from build123d import *

# Parameters (mm, degrees)
F1_DEPTH = 130
F2_R     = 6
F3_DEPTH = 5.001
F4_R     = 5
F5_DEPTH = 111.001


with BuildPart() as f1:
    # F0 (on Top) → F1 (new body)
    with BuildSketch(Plane.XY):
        with BuildLine():
            Line((17.922193, 92.008901), (-54.077807, 92.008901))
            Line((-54.077807, 92.008901), (-54.077807, 87.008901))
            Line((-54.077807, 87.008901), (14.922193, 87.008901))
            ThreePointArc((14.922193, 87.008901), (17.043514, 86.130221), (17.922193, 84.008901))
            Line((17.922193, 84.008901), (17.922193, -10.991095))
            ThreePointArc((17.922193, -10.991095), (17.043514, -13.112415), (14.922193, -13.991095))
            Line((14.922193, -13.991095), (-54.077807, -13.991095))
            Line((-54.077807, -13.991095), (-54.077807, -18.991099))
            Line((-54.077807, -18.991099), (17.922193, -18.991099))
            ThreePointArc((17.922193, -18.991099), (21.457727, -17.526633), (22.922193, -13.991099))
            Line((22.922193, -13.991099), (22.922193, 87.008901))
            ThreePointArc((22.922193, 87.008901), (21.457727, 90.544435), (17.922193, 92.008901))
        make_face()
    extrude(amount=F1_DEPTH)

    # F2 (on face) → F3 (cut, through all)
    with BuildSketch(Plane(origin=(17.922193, 0, 0), x_dir=(0, -1, 0), z_dir=(-1, 0, 0))):
        with Locations((-15.887585, 105)):
            Circle(F2_R)
        with Locations((-36.508901, 25)):
            Circle(F2_R)
        with Locations((-58.008901, 105)):
            Circle(F2_R)
    extrude(amount=-F3_DEPTH, mode=Mode.SUBTRACT)

    # F4 (on face) → F5 (cut, through all)
    with BuildSketch(Plane(origin=(0, 92.008901, 0), x_dir=(-1, 0, 0), z_dir=(0, 1, 0))):
        with Locations((39.077807, 25)):
            Circle(F4_R)
        with Locations((4.077807, 25)):
            Circle(F4_R)
        Polygon((12.077807, 75), (54.077807, 30), (54.077807, 130), (-17.922193, 130), (-17.922193, 75), align=None)
    extrude(amount=-F5_DEPTH, mode=Mode.SUBTRACT)


solid = f1.part
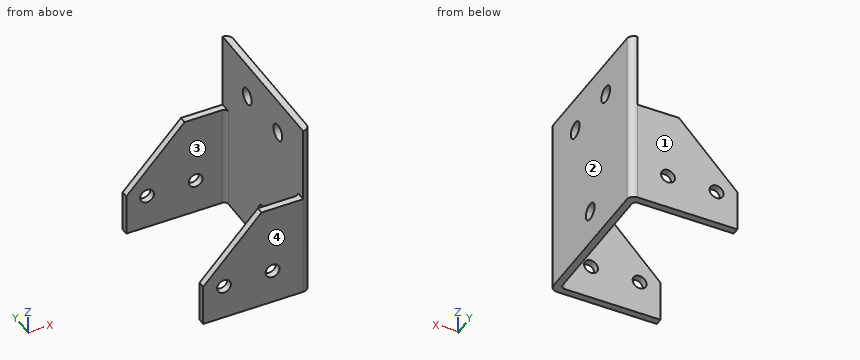
Could you check a few things on this model? Use its own coordinates, in mm. Face numbers are marked on the shaded views. Coordinates: 2 decimals unless noted, no trailing zeros. Write each loop counter-clockwise with the first axis right and the second up, starting at its lowest first coordinate (ties: lowest second). Pieces come first, ordered by that corner, then holes. Notation, with made-up numbers: M -15,58.5 L 43,58.5 A16 cw 43,67.5 Z; hole C 32,-7.5 d1. An arc over 180 degrees is marked long. One line per question, with ' | ' between items.
1) If we mould it in two halves opening along Y, with no side actions, what happens to the marked faces 1, 2, 3 and 4? For each: released by +Y, released by -Y, zero draft, split by the parting line, or undercut.
Checks:
face 1: released by +Y | face 2: zero draft | face 3: undercut | face 4: released by -Y
2) Imagine slicing it at A-A, the plane x = 7. Write out the boundary of the cut face in (y, z), and give its area (3 significant figures).
Checks:
outline: M -18.99,0 L -13.99,0 L -13.99,75 L -18.99,75 Z; M 87.01,0 L 92.01,0 L 92.01,75 L 87.01,75 Z | area: 750 mm²
3) I need wall thicknesses on probe 1 along Y at (x, z) = (2.5, 51.5); probe 2 along X at (y, z) = (-12, 121); probe 3 along X at (y, z) = (86, 52). Which ranges of each line are inside material? Lowest first, please. Write a range as [from, to].
Checks:
probe 1: [-18.99, -13.99], [87.01, 92.01] | probe 2: [17.92, 22.92] | probe 3: [17.17, 22.92]
4) Imagine slicing it at C-C, the plane z = 105. Write out the boundary of the cut face in (x, y), and give its area (3 significant figures).
Checks:
outline: M 17.92,-18.99 A5 ccw 22.92,-13.99 L 22.92,9.89 L 17.92,9.89 Z; M 17.92,21.89 L 22.92,21.89 L 22.92,52.01 L 17.92,52.01 Z; M 17.92,64.01 L 22.92,64.01 L 22.92,87.01 A5 ccw 17.92,92.01 Z | area: 424 mm²
5) Imagine slicing it at D-D, the plane x = -41. Write out the boundary of the cut face in (y, z), and give its area (3 significant figures).
Checks:
outline: M -18.99,0 L -13.99,0 L -13.99,20.38 L -18.99,20.38 Z; M -18.99,29.62 L -13.99,29.62 L -13.99,44.01 L -18.99,44.01 Z; M 87.01,0 L 92.01,0 L 92.01,20.38 L 87.01,20.38 Z; M 87.01,29.62 L 92.01,29.62 L 92.01,44.01 L 87.01,44.01 Z | area: 348 mm²
6) For pin 1 Ø9 at (x, z) = (-39.08, 25) entering from +Y; pin 2 Ø4 at (y, z) = (75, 20.5) entering from -X; pin 3 Ø4 at (x, y) = (9.5, 86.5) entering from +Z, each with a flat end and sliding along its axis, tell me the tip position at first contact or that it passes through.
Checks:
pin 1: through | pin 2: x = 17.92 | pin 3: z = 75
7) Imagine slicing it at B-B, the plane z = 25. Give the number of separate pieces and of enclosed holes in the cut face, and give its area (3 significant figures).
Checks:
separate pieces: 6 | enclosed holes: 0 | area: 1,010 mm²
